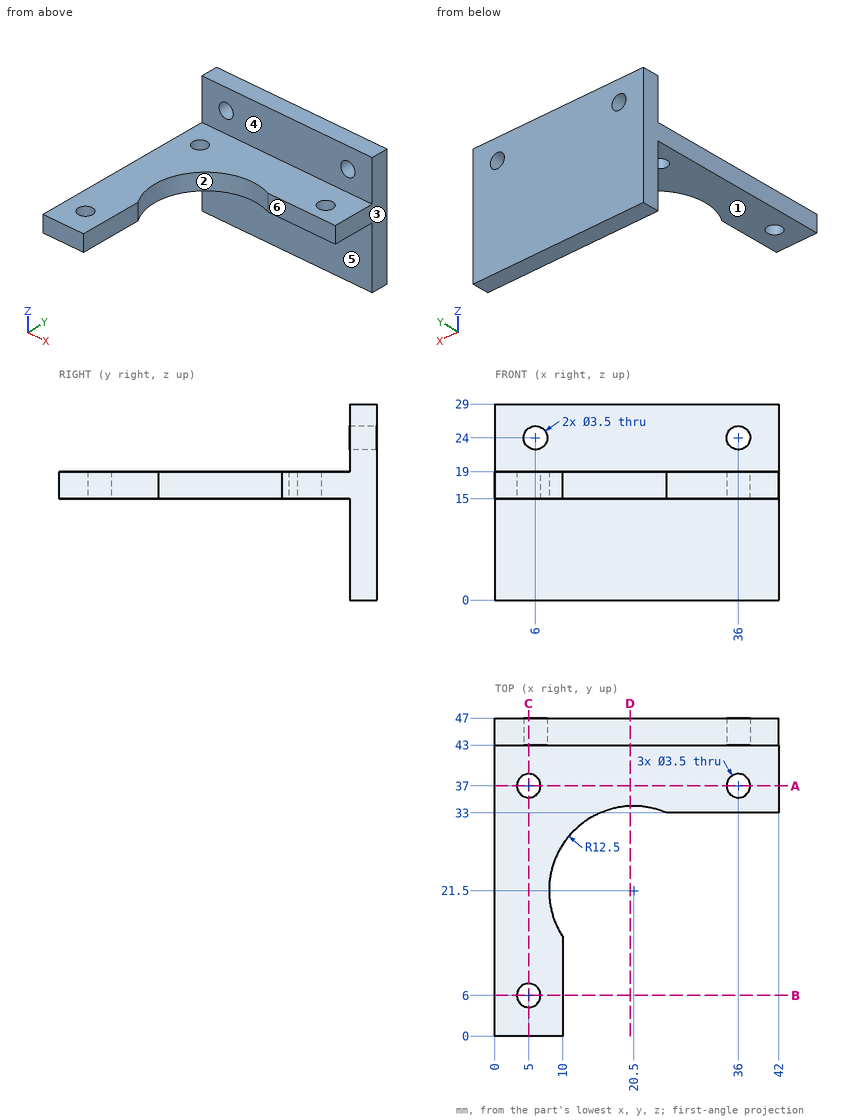
Check sheet for the drawn part. Datum: minimum x, y, z corner. Units: mm. A direction names the side the tool comes from. Coordinates: 2 decimals unless noted, no trailing zeros. Order: outer loops, then holes, each group sorted by start corner. A loop starts at its lowest first (then second) coordinate and runs counter-clockwise, first axis right, second up. Notation, with made-up numbers: (75, 10) -> (121, 10) arc R31 ccw to (121, 47) -> close; hole circle Ø9 at (-24.5, 24). An arc over 180 degrees is marked (long way). Use a Markdown table: item, result. Add a question column.
1. Material ranges on L1, parallel to Y at x = 5, z = 15.95; L2, parallel to X at y = 44.9, z = 24; L3, parallel to Y at x = 22.5, z = 1.25, recorded low to high.
2. Go/stop test with flat-tipped pins: pin 1 Ø6 at (x, z) = (20.5, 4.5) entering from -Y; pin 2 Ø5 at (x, y) = (8, 23) entering from +Z; pin 3 Ø5 at (y, z) = (14, 20) entering from +X. Record where each tip stops, or that it passes through.
3. Mould release check, pull along X, two halves, no side actions. Record for the marked faces 1, 2 and 3: pulls with the +X half, pulls with the -X half, needs draft (parallel to the pull), parting line crosses it, or undercut.
4. Cross-section at A-A (y = 37). Enter the section's corners in (x, z).
5. Cross-section at C-C (x = 5). Enter the section's corners in (y, z).
6. Cross-section at B-B (y = 6). Enter the section's corners in (x, z).
7. Cross-section at D-D (x = 20). Enter the section's corners in (y, z), and give its area (3 significant figures).
8. Set-up check for the marked faces 4, 5 and 6: record each of +Z, -Z, +X, -X, +Y, -Y from which the full face is reachable in a straight line by a thin tool's end or side.
Filled sheet:
| question | item | result |
|---|---|---|
| 1 | L1 | 0 to 4.25, 7.75 to 35.25, 38.75 to 47 |
| 1 | L2 | 0 to 4.25, 7.75 to 34.25, 37.75 to 42 |
| 1 | L3 | 43 to 47 |
| 2 | pin 1 | y = 43 |
| 2 | pin 2 | z = 19 |
| 2 | pin 3 | x = 10 |
| 3 | face 1 | needs draft |
| 3 | face 2 | undercut |
| 3 | face 3 | pulls with the +X half |
| 4 | outline | (0, 15) -> (3.25, 15) -> (3.25, 19) -> (0, 19) -> close; (6.75, 15) -> (34.25, 15) -> (34.25, 19) -> (6.75, 19) -> close; (37.75, 15) -> (42, 15) -> (42, 19) -> (37.75, 19) -> close |
| 5 | outline | (0, 15) -> (4.25, 15) -> (4.25, 19) -> (0, 19) -> close; (7.75, 15) -> (35.25, 15) -> (35.25, 19) -> (7.75, 19) -> close; (38.75, 15) -> (43, 15) -> (43, 0) -> (47, 0) -> (47, 22.56) -> (43, 22.56) -> (43, 19) -> (38.75, 19) -> close; (43, 25.44) -> (47, 25.44) -> (47, 29) -> (43, 29) -> close |
| 6 | outline | (0, 15) -> (3.25, 15) -> (3.25, 19) -> (0, 19) -> close; (6.75, 15) -> (10, 15) -> (10, 19) -> (6.75, 19) -> close |
| 7 | outline | (33.99, 15) -> (43, 15) -> (43, 0) -> (47, 0) -> (47, 29) -> (43, 29) -> (43, 19) -> (33.99, 19) -> close |
| 7 | area | 152 mm2 |
| 8 | face 4 | +Z, +X, -X, -Y |
| 8 | face 5 | -Z, +X, -X, -Y |
| 8 | face 6 | +Z, -Z, +X, -Y |
